from build123d import *

# Parameters (mm, degrees)
SKETCH1_W           = 33
SKETCH1_H           = 28
BOSS_EXTRUDE1_DEPTH = 46
CUT_EXTRUDE1_DEPTH  = 59.318093247
CUT_EXTRUDE2_START  = -3
CUT_EXTRUDE2_DEPTH  = 27
FILLET1_R           = 12.5
FILLET2_R           = 16.5
FILLET3_R           = 6
SKETCH4_W           = 13
SKETCH4_H           = 23
CUT_EXTRUDE3_DEPTH  = 9
SKETCH5_R           = 6.5
CUT_EXTRUDE4_DEPTH  = 56.592265809
SKETCH6_R           = 1
CUT_EXTRUDE5_DEPTH  = 8
SKETCH7_R           = 1.3
SKETCH7_R_2         = 2.5
CUT_EXTRUDE6_DEPTH  = 2.5


with BuildPart() as part:
    # Sketch1 → Boss-Extrude1 (new body)
    with BuildSketch(Plane.XY):
        Rectangle(SKETCH1_W, SKETCH1_H)
    extrude(amount=BOSS_EXTRUDE1_DEPTH)

    # Sketch2 → Cut-Extrude1 (cut, through all)
    with BuildSketch(Plane(origin=(16.5, 0, 0), x_dir=(0, 0, -1), z_dir=(1, 0, 0))):
        with BuildLine():
            Line((-46, 2), (-46, -14))
            Line((-46, -14), (-5, -14))
            add(Edge.make_bspline(
                [(-5, -14), (-24.445807758, -2.434726237), (-46, 2)],
                knots=[0, 0, 0, 1, 1, 1], degree=2))
        make_face()
    extrude(amount=-CUT_EXTRUDE1_DEPTH, mode=Mode.SUBTRACT)

    # Sketch3 → Cut-Extrude2 (cut)
    with BuildSketch(Plane(origin=(16.5, 0, 0), x_dir=(0, 0, -1), z_dir=(1, 0, 0)).offset(CUT_EXTRUDE2_START)):
        with BuildLine():
            Line((-5, -14), (-2.5, -14))
            Line((-2.5, -14), (-2.5, 3.5))
            Line((-2.5, 3.5), (-40.5, 3.5))
            Line((-40.5, 3.5), (-40.5, 0.743693735))
            add(Edge.make_bspline(
                [(-5, -14), (-21.949128929, -3.919610512), (-40.5, 0.743693735)],
                knots=[0, 0, 0, 1, 1, 1], degree=2))
        make_face()
    extrude(amount=-CUT_EXTRUDE2_DEPTH, mode=Mode.SUBTRACT)

    # Fillet1
    fillet1_edges = [part.edges().sort_by_distance(p)[0] for p in [
        (13.5, 2.121846868, 40.5),
        (-13.5, 2.121846868, 40.5),
    ]]
    fillet(fillet1_edges, radius=FILLET1_R)

    # Fillet2
    fillet2_edges = [part.edges().sort_by_distance(p)[0] for p in [
        (16.5, 8, 46),
        (-16.5, 8, 46),
    ]]
    fillet(fillet2_edges, radius=FILLET2_R - 0.0001)  # a hair under: the kernel refuses the full size

    # Fillet3
    fillet3_edges = [part.edges().sort_by_distance(p)[0] for p in [
        (-16.5, -14, 2.5),
        (16.5, -14, 2.5),
    ]]
    fillet(fillet3_edges, radius=FILLET3_R)

    # Sketch4 → Cut-Extrude3 (cut)
    with BuildSketch(Plane.XZ.offset(-3.5)):
        with Locations((0, 20.5)):
            Rectangle(SKETCH4_W, SKETCH4_H)
    extrude(amount=-CUT_EXTRUDE3_DEPTH, mode=Mode.SUBTRACT)

    # Sketch5 → Cut-Extrude4 (cut, through all)
    with BuildSketch(Plane.XZ.offset(-12.5)):
        with Locations((0, 25.5)):
            Circle(SKETCH5_R)
    extrude(amount=-CUT_EXTRUDE4_DEPTH, mode=Mode.SUBTRACT)

    # Sketch6 → Cut-Extrude5 (cut)
    with BuildSketch(Plane.XZ.offset(-3.5)):
        with Locations((0, 34.3)):
            Circle(SKETCH6_R)
        with Locations((0, 6.7)):
            Circle(SKETCH6_R)
    extrude(amount=-CUT_EXTRUDE5_DEPTH, mode=Mode.SUBTRACT)

    # Sketch7 → Cut-Extrude6 (cut)
    with BuildSketch(Plane(origin=(0, 0, 0), x_dir=(-1, 0, 0), z_dir=(0, 0, -1))):
        with Locations((0.5, 0)):
            Circle(SKETCH7_R)
        with Locations((5, 0)):
            Circle(SKETCH7_R_2)
        with Locations((9.5, 0)):
            Circle(SKETCH7_R)
    extrude(amount=-CUT_EXTRUDE6_DEPTH, mode=Mode.SUBTRACT)


solid = part.part
CAD build for the part. Positions are in the model's coordinates, mm. A direction names the side the tool comes from. Round coordinates to 2 decimals unless told otherwise and drop trailing zeros. Write item = value, one per line. Start each with the question number.
(1) Pin check, flat tips, straight feed: P1, Ø5, axis at x = 3.5, z = 30.5, coming from the -Y side; P2, Ø15, axis at x = 0, z = 25.5, coming from the +Y side; P3, Ø0.6, axis at x = 0.5, z = 34.5, coming from the -Y side; P4, Ø5, axis at x = -6, y = -5, coming from the +Z side. Stop position of each tip, or through.
(2) Probe line 1 (Z direction, x = 0, y = 9); line 2 (X direction, y = 13.25, z = 25.5); line 3 (X direction, y = 0.5, z = 11). List the from-to ranges inside material, lowest first. Write a range as [from, to].
(3) Which spindle directions (+Z, -Z, +X, -X, +Y, -Y) get a long thin tool onto all of the face, cutting with end or side? Do faces 1 (the flat face through (0, -14, 1)), 2 (the cylindrical face through (-7.385, 0.751, 1.232)), 3 (the cylindrical face through (11.16, 1.63, 35.28)). Say none if no direction does.
(4) Cut at A-A, the plane y = 8.25. State how many separate pieces and enclosed holes the cut face has, then the cut area to 3 significant figures.
(5) Pull direction Z, two halves, no side cores. Call faces 4 (the cylindrical face through (-1.74, 0.39, 1.23)), 5 (the cylindrical face through (11.538, 7.681, 41.295)), 6 (the cylindrical face through (-0.846, 13.24, 31.945)): released by +Z, released by -Z, zero draft, split by the parting line, or undercut.
Model answer:
q1.P1 = 3.5
q1.P2 = 14
q1.P3 = 11.5
q1.P4 = 2.5
q2.line_1 = [0, 5.7], [7.7, 9], [32, 33.3], [35.3, 46]
q2.line_2 = [-16.5, -6.5], [6.5, 16.5]
q2.line_3 = [-16.5, -13.5], [13.5, 16.5]
q3.face_1 = +Z, -Z, +X, -X, -Y
q3.face_2 = -Z
q3.face_3 = -Y
q4.separate_pieces = 1
q4.enclosed_holes = 3
q4.area = 1,100 mm2
q5.face_4 = zero draft
q5.face_5 = released by +Z
q5.face_6 = undercut
